Build history of the part. All positions in model axes, mm. A direction names the side the tool comes from. Round coordinates to 2 decimals unless told otherwise and drop trailing zeros. Write each loop counter-clockwise with the first axis right and the second up, starting at its lowest first coordinate (ties: lowest second). Pieces come first, ordered by that corner, then holes. Notation, with made-up numbers: (7, -8) -> (28, -8) arc R19 ccw to (28, 25) -> close; hole circle Ø5 at (7.5, 79). An arc over 180 degrees is marked (long way). Return JSON: item names as keys, results as strings.
from build123d import *

# Parameters (mm, degrees)
SKETCH1_W           = 52
SKETCH1_H           = 52.5
SKETCH1_R           = 2
SKETCH1_R_2         = 13.25
BOSS_EXTRUDE1_DEPTH = 2
SKETCH3_W           = 52
SKETCH3_H           = 2
BOSS_EXTRUDE3_DEPTH = 48
FILLET1_R           = 1.5
FILLET2_R           = 2.5
SKETCH7_R           = 7
SKETCH7_R_2         = 2
CUT_EXTRUDE1_DEPTH  = 76.909485573


with BuildPart() as part:
    # Sketch1 → Boss-Extrude1 (new body)
    with BuildSketch(Plane(origin=(0, 0, 0), x_dir=(0, 0, -1), z_dir=(1, 0, 0))):
        with Locations((0, 3.75)):
            Rectangle(SKETCH1_W, SKETCH1_H)
        with Locations((0, 17.5)):
            Circle(SKETCH1_R, mode=Mode.SUBTRACT)
        with Locations((17.5, 0)):
            Circle(SKETCH1_R, mode=Mode.SUBTRACT)
        with Locations((0, -17.5)):
            Circle(SKETCH1_R, mode=Mode.SUBTRACT)
        with Locations((-17.5, 0)):
            Circle(SKETCH1_R, mode=Mode.SUBTRACT)
        Circle(SKETCH1_R_2, mode=Mode.SUBTRACT)
    extrude(amount=BOSS_EXTRUDE1_DEPTH)

    # Sketch3 → Boss-Extrude3 (add)
    with BuildSketch(Plane(origin=(2, 0, 0), x_dir=(0, 0, -1), z_dir=(1, 0, 0))):
        with Locations((0, 31)):
            Rectangle(SKETCH3_W, SKETCH3_H)
    extrude(amount=-BOSS_EXTRUDE3_DEPTH)

    # Fillet1
    fillet1_edges = [part.edges().sort_by_distance(p)[0] for p in [
        (0, 30, 0),
    ]]
    fillet(fillet1_edges, radius=FILLET1_R)

    # Fillet2
    fillet2_edges = [part.edges().sort_by_distance(p)[0] for p in [
        (2, 32, 0),
    ]]
    fillet(fillet2_edges, radius=FILLET2_R)

    # Sketch7 → Cut-Extrude1 (cut, through all)
    with BuildSketch(Plane(origin=(0, 32, 0), x_dir=(1, 0, 0), z_dir=(0, 1, 0))):
        with Locations(Location((-23.25, 0, 0), (0, 0, 270))):
            Circle(SKETCH7_R)
        with Locations(Location((-39.25, 16, 0), (0, 0, 270))):
            Circle(SKETCH7_R_2)
        with Locations(Location((-31.25, 16, 0), (0, 0, 270))):
            Circle(SKETCH7_R_2)
        with Locations(Location((-23.25, 16, 0), (0, 0, 270))):
            Circle(SKETCH7_R_2)
        with Locations(Location((-15.25, 16, 0), (0, 0, 270))):
            Circle(SKETCH7_R_2)
        with Locations(Location((-7.25, 16, 0), (0, 0, 270))):
            Circle(SKETCH7_R_2)
        with Locations(Location((-31.25, 8, 0), (0, 0, 270))):
            Circle(SKETCH7_R_2)
        with Locations(Location((-15.25, 8, 0), (0, 0, 270))):
            Circle(SKETCH7_R_2)
        with Locations(Location((-7.25, 8, 0), (0, 0, 270))):
            Circle(SKETCH7_R_2)
        with Locations(Location((-7.25, 0, 0), (0, 0, 270))):
            Circle(SKETCH7_R_2)
        with Locations(Location((-31.25, -8, 0), (0, 0, 270))):
            Circle(SKETCH7_R_2)
        with Locations(Location((-15.25, -8, 0), (0, 0, 270))):
            Circle(SKETCH7_R_2)
        with Locations(Location((-7.25, -8, 0), (0, 0, 270))):
            Circle(SKETCH7_R_2)
        with Locations(Location((-31.25, -16, 0), (0, 0, 270))):
            Circle(SKETCH7_R_2)
        with Locations(Location((-23.25, -16, 0), (0, 0, 270))):
            Circle(SKETCH7_R_2)
        with Locations(Location((-15.25, -16, 0), (0, 0, 270))):
            Circle(SKETCH7_R_2)
        with Locations(Location((-7.25, -16, 0), (0, 0, 270))):
            Circle(SKETCH7_R_2)
        with Locations(Location((-39.25, 8, 0), (0, 0, 270))):
            Circle(SKETCH7_R_2)
        with Locations(Location((-39.25, 0, 0), (0, 0, 270))):
            Circle(SKETCH7_R_2)
        with Locations(Location((-39.25, -8, 0), (0, 0, 270))):
            Circle(SKETCH7_R_2)
        with Locations(Location((-39.25, -16, 0), (0, 0, 270))):
            Circle(SKETCH7_R_2)
    extrude(amount=-CUT_EXTRUDE1_DEPTH, mode=Mode.SUBTRACT)


solid = part.part
Q1. Saw through at D-D on y = 17.5. List the corners of the cut face in (x, z).
Verdict:
{"outline": "(0, -26) -> (2, -26) -> (2, -2) -> (0, -2) -> close; (0, 2) -> (2, 2) -> (2, 26) -> (0, 26) -> close"}
Q2. Pin check, flat tips, straight feed: pin 1 Ø4.5 at (x, z) = (-39.25, 0) entering from -Y; pin 2 Ø12 at (y, z) = (-13, 19) entering from -X. Stop position of each tip, or through.
Verdict:
{"pin 1": "stops at y = 30", "pin 2": "stops at x = 0"}
Q3. Saw through at A-A on y = 0. List the corners of the cut face in (x, z), then the cut area to 3 significant figures.
Verdict:
{"outline": "(0, -26) -> (2, -26) -> (2, -19.5) -> (0, -19.5) -> close; (0, -15.5) -> (2, -15.5) -> (2, -13.25) -> (0, -13.25) -> close; (0, 13.25) -> (2, 13.25) -> (2, 15.5) -> (0, 15.5) -> close; (0, 19.5) -> (2, 19.5) -> (2, 26) -> (0, 26) -> close", "area": "35.0 mm²"}
Q4. Wall check: L1, parallel to X at y = -2, z = -18.5; L2, parallel to Y at x = -15, z = -2; L3, parallel to X at y = 30.9, z = -16. Give the ranges that are in metal, low to high.
Verdict:
{"L1": "x = 0 to 2", "L2": "y = 30 to 32", "L3": "x = -46 to -41.25, -37.25 to -33.25, -29.25 to -25.25, -21.25 to -17.25, -13.25 to -9.25, -5.25 to 1.57"}
Q5. Saw through at B-B on x = -31.25. List the corners of the cut face in (y, z), then the cut area to 3 significant figures.
Verdict:
{"outline": "(30, -26) -> (32, -26) -> (32, -18) -> (30, -18) -> close; (30, -14) -> (32, -14) -> (32, -10) -> (30, -10) -> close; (30, -6) -> (32, -6) -> (32, 6) -> (30, 6) -> close; (30, 10) -> (32, 10) -> (32, 14) -> (30, 14) -> close; (30, 18) -> (32, 18) -> (32, 26) -> (30, 26) -> close", "area": "72.0 mm²"}
Q6. Two-plate mould, pull along X, no slides. Class faces 1 (the cylindrical face through (1.248, 31.287, -0.364)), 2 (the cylindrical face through (-21.267, 31.014, 15.74)), 3 (the flat face through (1, 17, -26)): +X half, -X half, draft (parallel to the pull), parting line (faces both ways), or undercut.
Verdict:
{"face 1": "+X half", "face 2": "undercut", "face 3": "draft"}
Q7. Saw through at C-C on x = -23.25. List the corners of the cut face in (y, z), then the cut area to 3 significant figures.
Verdict:
{"outline": "(30, -26) -> (32, -26) -> (32, -18) -> (30, -18) -> close; (30, -14) -> (32, -14) -> (32, -7) -> (30, -7) -> close; (30, 7) -> (32, 7) -> (32, 14) -> (30, 14) -> close; (30, 18) -> (32, 18) -> (32, 26) -> (30, 26) -> close", "area": "60.0 mm²"}
Q8. 3-axis set-ups, long thin cutter, end or side, ignore diameter. For faces 4 (the cylindrical face through (-33.202, 31.014, -16.434)), 5 (the flat face through (-18, 30, 6)): which of +Z, -Z, +X, -X, +Y, -Y reach the whole face in a straight line?
Verdict:
{"face 4": "+Y, -Y", "face 5": "+Z, -Z, -X, -Y"}
